```python
from build123d import *

# Parameters (mm, degrees)
F0_W     = 388
F0_H     = 682
F1_DEPTH = 12
F2_W     = 6
F2_H     = 682
F3_DEPTH = 6
F4_W     = 382
F4_H     = 6
F5_DEPTH = 6
F6_W     = 6
F6_H     = 676
F7_DEPTH = 6
F8_W     = 376
F8_H     = 6
F9_DEPTH = 6


with BuildPart() as f1:
    # F0 (on Front) → F1 (new body)
    with BuildSketch(Plane.XZ):
        Rectangle(F0_W, F0_H)
    extrude(amount=F1_DEPTH)

    # F2 (on face) → F3 (cut)
    with BuildSketch(Plane(origin=(0, 0, 0), x_dir=(-1, 0, 0), z_dir=(0, 1, 0))):
        with Locations((191, 0)):
            Rectangle(F2_W, F2_H)
    extrude(amount=-F3_DEPTH, mode=Mode.SUBTRACT)

    # F4 (on face) → F5 (cut)
    with BuildSketch(Plane(origin=(0, 0, 0), x_dir=(-1, 0, 0), z_dir=(0, 1, 0))):
        with Locations((-3, -338)):
            Rectangle(F4_W, F4_H)
    extrude(amount=-F5_DEPTH, mode=Mode.SUBTRACT)

    # F6 (on face) → F7 (cut)
    with BuildSketch(Plane(origin=(0, 0, 0), x_dir=(-1, 0, 0), z_dir=(0, 1, 0))):
        with Locations((-191, 3)):
            Rectangle(F6_W, F6_H)
    extrude(amount=-F7_DEPTH, mode=Mode.SUBTRACT)

    # F8 (on face) → F9 (cut)
    with BuildSketch(Plane(origin=(0, 0, 0), x_dir=(-1, 0, 0), z_dir=(0, 1, 0))):
        with Locations((0, 83)):
            Rectangle(F8_W, F8_H)
    extrude(amount=-F9_DEPTH, mode=Mode.SUBTRACT)


solid = f1.part
```
Here's how the part is built. I have some questions about the finished solid (model axes, mm). Give positions to 0.01 mm unless a question says otherwise; leave off trailing zeros. Write each loop counter-clockwise with the first axis right and the second up, starting at its lowest first coordinate (ties: lowest second). Pieces come first, ordered by that corner, then holes. Notation, with made-up numbers: (87, 75.5) -> (101, 75.5) arc R27 ccw to (101, 104.5) -> close; hole circle Ø10 at (-27.5, -31). An arc over 180 degrees is marked (long way). Write each question's results on one line, items separated by ' | '.
Item 1: If I drill on L1, parallel to Z at x = 28.5, y = -5.5; L2, parallel to X at y = -1, z = -226, over which ranges is the centre line in solid material (lowest first)?
Output:
L1: z = -335 to 80, 86 to 341 | L2: x = -188 to 188
Item 2: Suppose I cut it at A-A on y = -4. Write out the boundary of the cut face in (x, z), plus the area to 3 significant figures.
Output:
outline: (-188, -335) -> (188, -335) -> (188, 80) -> (-188, 80) -> close; (-188, 86) -> (188, 86) -> (188, 341) -> (-188, 341) -> close | area: 252,000 mm^2
Item 3: Suppose I cut it at B-B on z = -215. Write out the boundary of the cut face in (x, y), plus the area to 3 significant figures.
Output:
outline: (-194, -12) -> (194, -12) -> (194, -6) -> (188, -6) -> (188, 0) -> (-188, 0) -> (-188, -6) -> (-194, -6) -> close | area: 4,580 mm^2
Item 4: For pin 1 Ø1.8 at (y, z) = (-2.5, -162.5) entering from +X; pin 2 Ø1.8 at (y, z) = (-4.5, 232) entering from -X; pin 3 Ø3 at (x, y) = (71, -3) entering from -Z, each with a flat end and sliding along its axis, tell me the tip position at first contact or that it passes through.
Output:
pin 1: stops at x = 188 | pin 2: stops at x = -188 | pin 3: stops at z = -335
Item 5: We'd pull the mould along Z, two halves only. Please class faces 1 (the face through (-3, -6, 341)), 2 (the face through (-3, -12, 5)): pulls with the +Z half, pulls with the -Z half, needs draft (parallel to the pull), parting line crosses it, or undercut.
Output:
face 1: pulls with the +Z half | face 2: needs draft
